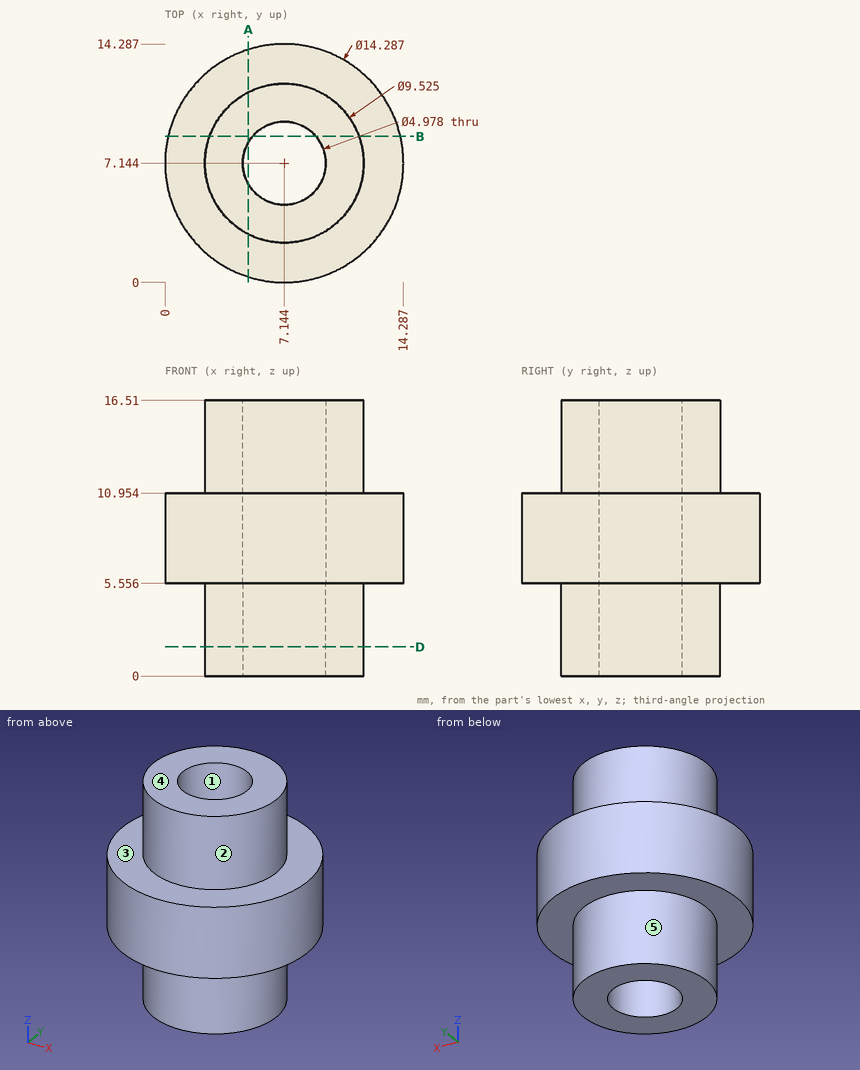
Source: three-view drawing plus pictorial views. Frame: mm from the lowest corner of the part. A direction names the side the tool comes from. Give positions to 0.01 mm unless a question says otherwise; leave off trailing zeros. Loops run counter-clockwise (first coordinate to the right, second up) from the corner with the lowest first, then second, coordinate; pieces in that order, holes last. Notation, with made-up numbers: (55.5, -11.5) -> (85.5, -11.5) arc R35 cw to (85.5, 24.5) -> close; hole circle Ø9 at (69.5, 0). An arc over 180 degrees is marked (long way). Put each result on its own line as item: value. Start each with the question number.
1) Contact query for flat-ended pins moving along their axis: P1, Ø4.5, axis at x = 7, y = 7.5, coming from the -Z side; P2, Ø4, axis at x = 5.5, z = 2.5, coming from the +Y side; P3, Ø8, axis at x = 2.5, z = 7.5, coming from the +Y side; P4, Ø1.5, axis at y = 12, z = 3.5, coming from the -X side. Output: stop coordinate, or through.
2) Cut plane A-A (x = 5). Return loops of the section in (y, z).
3) Cut plane D-D (z = 1.75). Return loops of the section in (x, y) (1 decimal), then the cut area to 3 significant figures.
4) Draft query along Y for the marked faces 1, 2 and 3. Return one class per face: released by +Y, released by -Y, zero draft, split by the parting line, or undercut.
5) Reachability of the marked faces 4 and 5 from +Z, -Z, +X, -X, +Y, -Y: full face, straight path, thin tool, end or side. Return the list, or none.
6) Cut plane B-B (y = 8.75). Return loops of the section in (x, z) (1 decimal).
7) Material intervals for probe 1 along X at (y, z) = (7.25, 13.25) (1 decimal); probe 2 along Z at (x, y) = (13, 4); probe 3 along Y at (x, z) = (9.25, 2.5) (1 decimal), sorted ascending.
Results are:
1. P1: stops at z = 0
1. P2: stops at y = 11.91
1. P3: stops at y = 14.26
1. P4: stops at x = 4.73
2. outline: (0.33, 5.56) -> (2.89, 5.56) -> (2.89, 0) -> (5.88, 0) -> (5.88, 16.51) -> (2.89, 16.51) -> (2.89, 10.95) -> (0.33, 10.95) -> close; (8.41, 0) -> (11.4, 0) -> (11.4, 5.56) -> (13.96, 5.56) -> (13.96, 10.95) -> (11.4, 10.95) -> (11.4, 16.51) -> (8.41, 16.51) -> close
3. outline: circle Ø9.5 at (7.1, 7.1); hole circle Ø5 at (7.1, 7.1)
3. area: 51.8 mm2
4. face 1: undercut
4. face 2: split by the parting line
4. face 3: zero draft
5. face 4: +Z, +X, -X, +Y, -Y
5. face 5: -Z
6. outline: (0.2, 5.6) -> (2.7, 5.6) -> (2.7, 0) -> (5.2, 0) -> (5.2, 16.5) -> (2.7, 16.5) -> (2.7, 11) -> (0.2, 11) -> close; (9, 0) -> (11.6, 0) -> (11.6, 5.6) -> (14.1, 5.6) -> (14.1, 11) -> (11.6, 11) -> (11.6, 16.5) -> (9, 16.5) -> close
7. probe 1: x = 2.4 to 4.7, 9.6 to 11.9
7. probe 2: z = 5.56 to 10.95
7. probe 3: y = 2.9 to 5.8, 8.5 to 11.4
